```python
from build123d import *

# Parameters (mm, degrees)
F0_W         = 78
F0_H         = 78
F1_DEPTH     = 86
F2_T         = -4
F4_DEPTH     = 24
F3_W         = 70
F3_H         = 20
F5_DEPTH     = 74
F6_W         = 78
F6_H         = 78
F6_W_2       = 74
F6_H_2       = 74
F7_DEPTH     = 20
F9_DEPTH     = 2
F10_R        = 3.99999
F11_R        = 4
F12_W        = 40
F12_H        = 2
F13_DEPTH    = 0.3
F14_T1_DEPTH = 43.5707142143
F15_T1_DEPTH = 43.5707142143


# Not quite as in the source:
# - a fillet or chamfer that OpenCascade refuses, or shapes differently, is made with other operations: its cross-section is extruded or revolved along the edge and cut away or added
# - a fillet or chamfer is up to 0.001 mm smaller than in the source, because OpenCascade refuses the exact size


with BuildPart() as f1:
    # F0 (on Top) → F1 (new body)
    with BuildSketch(Plane.XY):
        with Locations((-38.7419309749, 20.0862393249)):
            Rectangle(F0_W, F0_H)
    extrude(amount=F1_DEPTH)

    # F2
    f2_openings = [f1.faces().sort_by_distance(p)[0] for p in [
        (-38.741931, 20.086239, 86),
    ]]
    offset(amount=F2_T, openings=f2_openings)

    # F4 (add): a face of the model
    f4_faces = [f1.faces().sort_by_distance(p)[0] for p in [
        (-38.7419309749, 20.0862393249, 4),
    ]]
    extrude(f4_faces, amount=F4_DEPTH)

    # F3 (on face) → F5 (cut)
    with BuildSketch(Plane.XZ.offset(18.9137606751)):
        with Locations((-38.7419309749, 13)):
            Rectangle(F3_W, F3_H)
    extrude(amount=-F5_DEPTH, mode=Mode.SUBTRACT)

    # F6 (on face) → F7 (cut)
    with BuildSketch(Plane.XY.offset(86)):
        with Locations((-38.7419309749, 20.0862393249)):
            Rectangle(F6_W, F6_H)
        with Locations((-38.7419309749, 20.0862393249)):
            Rectangle(F6_W_2, F6_H_2, mode=Mode.SUBTRACT)
    extrude(amount=-F7_DEPTH, mode=Mode.SUBTRACT)

    # F8 (on face) → F9 (join)
    with BuildSketch(Plane.YZ.offset(-1.7419309749)):
        with BuildLine():
            Line((-6.9137606751, 66), (47.0862393249, 66))
            ThreePointArc((47.0862393249, 66), (20.0862393249, 73), (-6.9137606751, 66))
        make_face()
    extrude(amount=F9_DEPTH)

    # F10 (radius 4 in the source; OpenCascade refuses exactly that, so slightly less here)
    f10_edges = [f1.edges().sort_by_distance(p)[0] for p in [
        (-77.741931, -18.913761, 33),
        (0.258069, -18.913761, 33),
        (0.258069, 59.086239, 33),
        (-77.741931, 59.086239, 33),
    ]]
    fillet(f10_edges, radius=F10_R)

    # F11
    f11_edges = [f1.edges().sort_by_distance(p)[0] for p in [
        (-1.741931, -16.913761, 76),
        (-1.741931, 57.086239, 76),
        (-75.741931, -16.913761, 76),
        (-75.741931, 57.086239, 76),
    ]]
    fillet(f11_edges, radius=F11_R)

    # F12 (on face) → F13 (join)
    with BuildSketch(Plane.XZ.offset(16.9137606751)):
        with Locations((-38.7419309749, 76)):
            Rectangle(F12_W, F12_H)
    extrude(amount=F13_DEPTH)

    # F14: fillet of radius 1 on 1 edges, made by hand

    # F14_s2 → F14_t1 (cut)
    with BuildSketch(Plane.YZ.offset(-60.527288082)):
        with BuildLine():
            ThreePointArc((-16.9137606751, 77), (-17.1357151208, 76.6731554918), (-17.2137606751, 76.2858571571))
            Line((-17.2137606751, 76.2858571571), (-17.2137606751, 77))
            Line((-17.2137606751, 77), (-16.9137606751, 77))
        make_face()
    extrude(amount=F14_T1_DEPTH, mode=Mode.SUBTRACT)

    # F15: fillet of radius 1 on 1 edges, made by hand

    # F15_s2 → F15_t1 (cut)
    with BuildSketch(Plane.YZ.offset(-60.527288082)):
        with BuildLine():
            ThreePointArc((-16.9137606751, 75), (-17.1357151208, 75.3268445082), (-17.2137606751, 75.7141428429))
            Line((-17.2137606751, 75.7141428429), (-17.2137606751, 75))
            Line((-17.2137606751, 75), (-16.9137606751, 75))
        make_face()
    extrude(amount=F15_T1_DEPTH, mode=Mode.SUBTRACT)


solid = f1.part
```
Input: part model. Units: mm. Frame: model coordinates. A direction names the side the tool comes from. Give positions to 0.01 mm unless a question says otherwise; leave off trailing zeros. Order: outer loops, then holes, each group sorted by start corner. A loop starts at its lowest first (then second) coordinate and runs counter-clockwise, first axis right, second up. Notation, with made-up numbers: (-40, -29.5) - (-12, -29.5) arc R28 ccw to (-12, 1.5) - close; hole circle Ø10 at (50, -38.5). An arc over 180 degrees is marked (long way). Use a Markdown table: item, result.
(1) Section query C-C (x = -65.5). Output: boundary loops of the cut face in (y, z).
Computed values:
| item | result |
|---|---|
| outline | (-18.91, 0) - (59.09, 0) - (59.09, 66) - (57.09, 66) - (57.09, 86) - (55.09, 86) - (55.09, 28) - (-14.91, 28) - (-14.91, 86) - (-16.91, 86) - (-16.91, 66) - (-18.91, 66) - (-18.91, 23) - (55.09, 23) - (55.09, 3) - (-18.91, 3) - close |
(2) Draft query along Y for faces 1 (the cylindrical face through (-76.6, -17.71, 33.46)), 2 (the flat face through (-39, 21, 0)), 3 (the flat face through (-73.742, 20, 57)). Return one class per face: released by +Y, released by -Y, zero draft, split by the parting line, or undercut.
Computed values:
| item | result |
|---|---|
| face 1 | released by -Y |
| face 2 | zero draft |
| face 3 | undercut |
(3) Line query: line 1 (X direction, y = 35.5, z = 70); line 2 (Z direction, x = -18, y = 24); line 3 (X direction, y = -4, z = 15). Output: solid intervals per line, ascending. Write a range as from..to.
Computed values:
| item | result |
|---|---|
| line 1 | x = -75.74..-73.74, -3.74..0.26 |
| line 2 | z = 0..3, 23..28 |
| line 3 | x = -77.74..-73.74, -3.74..0.26 |
(4) Pin query (flat end, axial travel): pin 1 (16 mm diameter, centred on x = -28.5, z = 77.5, fed in from +Y); pin 2 (8 mm diameter, centred on x = -21, y = -6.5, fed in from -Z); pin 3 (6 mm diameter, centred on x = -54, z = 78, fed in from -Y); pin 4 (21 mm diameter, centred on x = -48, y = 35, fed in from +Z). Return the tip coordinate at first contact, or that it passes through.
Computed values:
| item | result |
|---|---|
| pin 1 | stops at y = 57.09 |
| pin 2 | stops at z = 0 |
| pin 3 | stops at y = -17.21 |
| pin 4 | stops at z = 28 |
(5) Access query for faces 4 (the flat face through (-39, 18, 3)), 5 (the cylindrical face through (-74.539, 55.946, 75.86)), 6 (the flat face through (-39, 55.086, 57)). Directions: +Z, -Z, +X, -X, +Y, -Y. A direction counts if a zero-diameter tool reaches every point of the face in a straight line with its end or side. Return the directions, or none.
Computed values:
| item | result |
|---|---|
| face 4 | -Y |
| face 5 | +Z, -X, +Y |
| face 6 | +Z |
(6) Section query A-A (y = -9). Output: boundary loops of the cut face in (x, z), then the cut area to 3 significant figures.
Computed values:
| item | result |
|---|---|
| outline | (-77.74, 0) - (0.26, 0) - (0.26, 66) - (-1.74, 66) - (-1.74, 86) - (-3.74, 86) - (-3.74, 28) - (-73.74, 28) - (-73.74, 86) - (-75.74, 86) - (-75.74, 66) - (-77.74, 66) - close; hole (-73.74, 3) - (-3.74, 3) - (-3.74, 23) - (-73.74, 23) - close |
| area | 1,170 mm2 |
(7) Section query B-B (z = 47). Output: boundary loops of the cut face in (x, y), then the cut area to 3 significant figures.
Computed values:
| item | result |
|---|---|
| outline | (-77.74, -14.91) arc R4 ccw to (-73.74, -18.91) - (-3.74, -18.91) arc R4 ccw to (0.26, -14.91) - (0.26, 55.09) arc R4 ccw to (-3.74, 59.09) - (-73.74, 59.09) arc R4 ccw to (-77.74, 55.09) - close; hole (-73.74, -14.91) - (-3.74, -14.91) - (-3.74, 55.09) - (-73.74, 55.09) - close |
| area | 1,170 mm2 |
